from build123d import *

# Parameters (mm, degrees)
ESTRUSIONE_ESTRUSIONE1_DEPTH = 190
TAGLIO_ESTRUSIONE1_DEPTH     = 190
TAGLIO_ESTRUSIONE2_DEPTH     = 191.053510761


with BuildPart() as part:
    # Schizzo1 → Estrusione-Estrusione1 (new body)
    with BuildSketch(Plane.XY):
        with BuildLine():
            ThreePointArc((2.184763914, -2.734375), (1.829579631, -2.841891076), (1.498123827, -2.675))
            ThreePointArc((1.498123827, -2.675), (0, -2), (-1.498123827, -2.675))
            ThreePointArc((-1.498123827, -2.675), (-1.829579631, -2.841891076), (-2.184763914, -2.734375))
            ThreePointArc((-2.184763914, -2.734375), (-3.5, 0), (-2.184763914, 2.734375))
            ThreePointArc((-2.184763914, 2.734375), (-1.829579631, 2.841891076), (-1.498123827, 2.675))
            ThreePointArc((-1.498123827, 2.675), (0, 2), (1.498123827, 2.675))
            ThreePointArc((1.498123827, 2.675), (1.829579631, 2.841891076), (2.184763914, 2.734375))
            ThreePointArc((2.184763914, 2.734375), (3.5, 0), (2.184763914, -2.734375))
        make_face()
        with BuildLine():
            ThreePointArc((-2.24718574, 1.9875), (-3, 0), (-2.24718574, -1.9875))
            ThreePointArc((-2.24718574, -1.9875), (-1.915729936, -2.154391076), (-1.560545653, -2.046875))
            ThreePointArc((-1.560545653, -2.046875), (0, -1.5), (1.560545653, -2.046875))
            ThreePointArc((1.560545653, -2.046875), (1.915729936, -2.154391076), (2.24718574, -1.9875))
            ThreePointArc((2.24718574, -1.9875), (3, 0), (2.24718574, 1.9875))
            ThreePointArc((2.24718574, 1.9875), (1.915729936, 2.154391076), (1.560545653, 2.046875))
            ThreePointArc((1.560545653, 2.046875), (0, 1.5), (-1.560545653, 2.046875))
            ThreePointArc((-1.560545653, 2.046875), (-1.915729936, 2.154391076), (-2.24718574, 1.9875))
        make_face(mode=Mode.SUBTRACT)
    extrude(amount=ESTRUSIONE_ESTRUSIONE1_DEPTH)

    # Schizzo2 → Taglio-Estrusione1 (cut)
    with BuildSketch(Plane(origin=(0, 0, 0), x_dir=(0, 0, -1), z_dir=(1, 0, 0))):
        with BuildLine():
            Line((-149.5, 0.5), (-130.5, 0.5))
            ThreePointArc((-130.5, 0.5), (-130, 0), (-130.5, -0.5))
            Line((-130.5, -0.5), (-149.5, -0.5))
            ThreePointArc((-149.5, -0.5), (-150, 0), (-149.5, 0.5))
        make_face()
    extrude(amount=-TAGLIO_ESTRUSIONE1_DEPTH, mode=Mode.SUBTRACT)

    # Schizzo3 → Taglio-Estrusione2 (cut, through all)
    with BuildSketch(Plane(origin=(0, 0, 0), x_dir=(0, 0, -1), z_dir=(1, 0, 0))):
        with BuildLine():
            Line((-12, 1), (-6, 1))
            ThreePointArc((-6, 1), (-5, 0), (-6, -1))
            Line((-6, -1), (-12, -1))
            ThreePointArc((-12, -1), (-13, 0), (-12, 1))
        make_face()
    extrude(amount=TAGLIO_ESTRUSIONE2_DEPTH, mode=Mode.SUBTRACT)


solid = part.part
Geometry: final body of the model. Coordinates: model frame, mm. A direction names the side the tool comes from. Give positions to 0.01 mm unless a question says otherwise; leave off trailing zeros. Loops run counter-clockwise (first coordinate to the right, second up) from the corner with the lowest first, then second, coordinate; pieces in that order, holes last. Notation, with made-up numbers: M 3,7 L 44,7 A25 cw 44,37 Z; hole C -5,59.25 d2. An arc over 180 degrees is marked long. Put each result on its own line as item: value. Start each with the question number.
1) Ray query, line 1 along X through (y, z) = (-1.7, 57); line 2 along Y through (x, z) = (-2.25, 31); line 3 along X through (y, z) = (-1.85, 43.5). Return the intervals inside material, ascending.
2) Cut plane A-A (z = 63.5). Output: boundary loops of the cut face in (x, y) (1 decimal).
3) Contact query for flat-ended pins moving along their axis: pin 1 (3 mm diameter, centred on x = -1.5, y = -1, fed in from +Z); pin 2 (2 mm diameter, centred on y = -1.5, z = 151.5, fed in from -X); pin 3 (0.6 mm diameter, centred on x = 3, z = 10, fed in from +Y). Output: stop coordinate, or through.
4) Pull-direction query (Y, two-part tool) for faces 1 (the cylindrical face through (-3.5, 0, 93.7)), 2 (the cylindrical face through (0, -1.5, 93.7)), 3 (the cylindrical face through (0, 2, 94)); classes: pulls with the +Y half, pulls with the -Y half, needs draft (parallel to the pull), parting line crosses it, or undercut.
5) Access query for faces 4 (the cylindrical face through (3.5, 0, 93.7)), 5 (the cylindrical face through (0, 1.5, 93.7)). Directions: +Z, -Z, +X, -X, +Y, -Y. A direction counts if a zero-diameter tool reaches every point of the face in a straight line with its end or side. Return the directions, or none.
Verdict:
1. line 1: -3.06 to -2.47, -0.98 to 0.98, 2.47 to 3.06
1. line 2: -2.68 to -1.98, 1.98 to 2.68
1. line 3: -2.97 to -2.36, -1.28 to 1.28, 2.36 to 2.97
2. outline: M -2.2,-2.7 A0.5 ccw -1.5,-2.7 A2 cw 1.5,-2.7 A0.5 ccw 2.2,-2.7 A3.5 ccw 2.2,2.7 A0.5 ccw 1.5,2.7 A2 cw -1.5,2.7 A0.5 ccw -2.2,2.7 A3.5 ccw Z; hole M -2.2,-2 A0.5 ccw -1.6,-2 A2.5 cw 1.6,-2 A0.5 ccw 2.2,-2 A3 ccw 2.2,2 A0.5 ccw 1.6,2 A2.5 cw -1.6,2 A0.5 ccw -2.2,2 A3 ccw Z
3. pin 1: z = 190
3. pin 2: x = -3.46
3. pin 3: y = 2.23
4. face 1: parting line crosses it
4. face 2: undercut
4. face 3: pulls with the +Y half
5. face 4: +Z, -Z, +X
5. face 5: +Z, -Z
